```python
from build123d import *

# Parameters (mm, degrees)
ESQUISSE1_W             = 1250
ESQUISSE1_H             = 800
BOSS_EXTRU_1_DEPTH      = 15
ESQUISSE2_W             = 1150
ESQUISSE2_H             = 700
ESQUISSE2_W_2           = 1126
ESQUISSE2_H_2           = 676
ENL_V_MAT_EXTRU_1_DEPTH = 7
ESQUISSE4_W             = 15
ESQUISSE4_H             = 676
ENL_V_MAT_EXTRU_2_DEPTH = 7


with BuildPart() as part:
    # Esquisse1 → Boss.-Extru.1 (new body)
    with BuildSketch(Plane.XY):
        Rectangle(ESQUISSE1_W, ESQUISSE1_H)
    extrude(amount=BOSS_EXTRU_1_DEPTH)

    # Esquisse2 → Enlèv. mat.-Extru.1 (cut)
    with BuildSketch(Plane.XY.offset(15)):
        Rectangle(ESQUISSE2_W, ESQUISSE2_H)
        Rectangle(ESQUISSE2_W_2, ESQUISSE2_H_2, mode=Mode.SUBTRACT)
    extrude(amount=-ENL_V_MAT_EXTRU_1_DEPTH, mode=Mode.SUBTRACT)

    # Esquisse4 → Enlèv. mat.-Extru.2 (cut)
    with BuildSketch(Plane.XY.offset(15)):
        with Locations((-355.5, 0)):
            Rectangle(ESQUISSE4_W, ESQUISSE4_H)
        with Locations((105.5, 0)):
            Rectangle(ESQUISSE4_W, ESQUISSE4_H)
    extrude(amount=-ENL_V_MAT_EXTRU_2_DEPTH, mode=Mode.SUBTRACT)


solid = part.part
```
The listing builds one solid part. Answer for the finished solid, in the listing's coordinates (mm). Give positions to 0.01 mm unless a question says otherwise; leave off trailing zeros. Write each loop counter-clockwise with the first axis right and the second up, starting at its lowest first coordinate (ties: lowest second). Pieces come first, ordered by that corner, then holes. Notation, with made-up numbers: (84.25, 39) -> (95.25, 39) arc R17 cw to (95.25, 45) -> close; hole circle Ø11 at (62, 37.5). An arc over 180 degrees is marked (long way). Use one line per item in the form item = value.
1) Straight lines are drawn through the part: probe 1 along X at (y, z) = (-291, 10); probe 2 along Y at (x, z) = (-141.5, 11); probe 3 along Z at (x, y) = (-573, 173). For each, find the intervals that lie inside material, in ascending order.
Result:
probe_1 = -625 to -575, -563 to -363, -348 to 98, 113 to 563, 575 to 625
probe_2 = -400 to -350, -338 to 338, 350 to 400
probe_3 = 0 to 8
2) Section B-B on y = 283.5 is taken. Write down the section's boundary in (x, z).
Result:
outline = (-625, 0) -> (625, 0) -> (625, 15) -> (575, 15) -> (575, 8) -> (563, 8) -> (563, 15) -> (113, 15) -> (113, 8) -> (98, 8) -> (98, 15) -> (-348, 15) -> (-348, 8) -> (-363, 8) -> (-363, 15) -> (-563, 15) -> (-563, 8) -> (-575, 8) -> (-575, 15) -> (-625, 15) -> close
3) Section A-A on z = 11 is taken. Write down the section's boundary in (x, y), plus the area to 3 significant figures.
Result:
outline = (-625, -400) -> (625, -400) -> (625, 400) -> (-625, 400) -> close; (-563, -338) -> (-363, -338) -> (-363, 338) -> (-563, 338) -> close; (-348, -338) -> (98, -338) -> (98, 338) -> (-348, 338) -> close; (113, -338) -> (563, -338) -> (563, 338) -> (113, 338) -> close; hole (-575, -350) -> (575, -350) -> (575, 350) -> (-575, 350) -> close
area = 936,000 mm²
4) For a pull along X with two mould halves and no side action, classify faces 1 (the flat face through (-49, -354, 15)), 2 (the flat face through (-3, 339, 8)) as +X half, -X half, draft (parallel to the pull), parting line (faces both ways), or undercut.
Result:
face_1 = draft
face_2 = undercut
